```python
from build123d import *

# Parameters (mm, degrees)
CROQUIS1_W              = 6.25
CROQUIS1_H              = 200
SALIENTE_EXTRUIR1_DEPTH = 3.125
CORTAR_EXTRUIR1_DEPTH   = 6.25
CROQUIS4_W              = 120
CROQUIS4_H              = 6.25
SALIENTE_EXTRUIR2_DEPTH = 6.25
SALIENTE_EXTRUIR3_DEPTH = 6.25
SALIENTE_EXTRUIR4_DEPTH = 6.25
CROQUIS10_R             = 1.5
CORTAR_EXTRUIR3_DEPTH   = 16.25


with BuildPart() as part:
    # Croquis1 → Saliente-Extruir1 (new, symmetric)
    with BuildSketch(Plane.XY):
        Rectangle(CROQUIS1_W, CROQUIS1_H)
    extrude(amount=SALIENTE_EXTRUIR1_DEPTH, both=True)

    # Croquis3 → Cortar-Extruir1 (cut)
    with BuildSketch(Plane.XY.offset(3.125)):
        Polygon((3.125, 100), (-3.125, 93.75), (-3.125, 100), align=None)
    extrude(amount=-CORTAR_EXTRUIR1_DEPTH, mode=Mode.SUBTRACT)

    # Croquis4 → Saliente-Extruir2 (add)
    with BuildSketch(Plane.XY.offset(3.125)):
        with Locations((-63.125, -96.875)):
            Rectangle(CROQUIS4_W, CROQUIS4_H)
    extrude(amount=-SALIENTE_EXTRUIR2_DEPTH)

    # Croquis7 → Saliente-Extruir3 (add)
    with BuildSketch(Plane.XY.offset(3.125)):
        Polygon((-123.125, -100), (3.125, 100), (-2.160090412, 103.336213323), (-130.516075072, -100), align=None)
    extrude(amount=-SALIENTE_EXTRUIR3_DEPTH)

    # Croquis9 → Saliente-Extruir4 (add)
    with BuildSketch(Plane.XY.offset(3.125)):
        Polygon((3.125, 100), (-2.160090412, 103.336213323), (3.125, 111.708633778), align=None)
    extrude(amount=-SALIENTE_EXTRUIR4_DEPTH)

    # Croquis10 → Cortar-Extruir3 (cut)
    with BuildSketch(Plane.XY.offset(3.125)):
        with Locations((0, -96.875)):
            Circle(CROQUIS10_R)
        with Locations((0, -89.375)):
            Circle(CROQUIS10_R)
        with Locations((-7.5, -96.875)):
            Circle(CROQUIS10_R)
    extrude(amount=-CORTAR_EXTRUIR3_DEPTH, mode=Mode.SUBTRACT)


solid = part.part
```
Geometry: final body of the model. Coordinates: model frame, mm. A direction names the side the tool comes from. Give positions to 0.01 mm unless a question says otherwise; leave off trailing zeros. Loops run counter-clockwise (first coordinate to the right, second up) from the corner with the lowest first, then second, coordinate; pieces in that order, holes last. Notation, with made-up numbers: (-18, 68) -> (21, 68) arc R16 cw to (21, 90) -> close; hole circle Ø3 at (6, 10). An arc over 180 degrees is marked (long way). Use one line per item in the form item = value.
Item 1: Section query B-B on y = 10.5. Output: boundary loops of the cut face in (x, z) (3 decimals), and give its area (3 significant figures).
A:
outline = (-60.763, -3.125) -> (-53.372, -3.125) -> (-53.372, 3.125) -> (-60.763, 3.125) -> close; (-3.125, -3.125) -> (3.125, -3.125) -> (3.125, 3.125) -> (-3.125, 3.125) -> close
area = 85.3 mm^2
Item 2: Section query A-A on x = -103.5. Output: boundary loops of the cut face in (y, z) (3 decimals).
A:
outline = (-100, -3.125) -> (-93.75, -3.125) -> (-93.75, 3.125) -> (-100, 3.125) -> close; (-68.911, -3.125) -> (-57.202, -3.125) -> (-57.202, 3.125) -> (-68.911, 3.125) -> close
Item 3: Section query C-C on z = 0.5. Output: boundary loops of the cut face in (x, y) (3 decimals), and give its area (3 significant figures).
A:
outline = (-130.516, -100) -> (3.125, -100) -> (3.125, 111.709) -> close; hole (-119.18, -93.75) -> (-3.125, -93.75) -> (-3.125, 90.099) -> close; hole circle Ø3 at (-7.5, -96.875); hole circle Ø3 at (0, -96.875); hole circle Ø3 at (0, -89.375)
area = 3,460 mm^2
Item 4: Pin query (flat end, axial travel): P1, Ø2.5, axis at x = -7.5, y = -96.875, coming from the -Z side; P2, Ø3, axis at x = -66, z = 1, coming from the +Y side. Return the tip coordinate at first contact, or that it passes through.
A:
P1 = through
P2 = 4.58
Item 5: Draft query along X for faces 3 (the face through (-68, -9, 3.125)), 4 (the face through (-3.125, -3, 0)), 5 (the face through (3.125, 7, 0)). Return one class per face: pulls with the +X half, pulls with the -X half, needs draft (parallel to the pull), parting line crosses it, or undercut.
A:
face_3 = needs draft
face_4 = undercut
face_5 = pulls with the +X half
Item 6: Access query for faces 1 (the face through (-61.965, -3.112, 0.044)), 2 (the face through (-65, -100, 0)). Directions: +Z, -Z, +X, -X, +Y, -Y. A direction counts if a zero-diameter tool reaches every point of the face in a straight line with its end or side. Return the directions, or none.
A:
face_1 = +Z, -Z
face_2 = +Z, -Z, +X, -X, -Y
Item 7: Line query: probe 1 along Y at (x, z) = (0, 1.5) (3 decimals); probe 2 along Y at (x, z) = (-7.5, 1.25) (3 decimals); probe 3 along X at (y, z) = (-46, 1.75) (1 decimal). Output: solid intervals per line, ascending.
A:
probe_1 = -100 to -98.375, -95.375 to -90.875, -87.875 to 106.758
probe_2 = -100 to -98.375, -95.375 to -93.75, 83.168 to 94.877
probe_3 = -96.4 to -89, -3.1 to 3.1
